Autodesk Inventor part; units mm, degrees
ref_plane "Work Plane1" through (90, 0, 0) normal (1, 0, 0) x (0, 1, 0)
ref_plane "Work Plane2" through (0, 0, 90) normal (0, 0, 1) x (1, 0, 0)
ref_plane "XZ Plane" through (0, 0, 0) normal (0, 1, 0) x (-1, 0, 0)
sketch "Sketch1" plane through (0, 0, 0) normal (0, 1, 0) x (-1, 0, 0)
  circle A0 centre (0, 0) radius 90
  dimension "d0" = 180
extrude "Extrusion1" add sketch "Sketch1" along normal blind 25
sketch "Sketch2" plane through (0, 25, 0) normal (0, 1, 0) x (1, 0, 0)
  line L0 (-30.75, 30.75) -> (30.75, 30.75)
  line L1 (30.75, 30.75) -> (30.75, -30.75)
  line L2 (30.75, -30.75) -> (-30.75, -30.75)
  line L3 (-30.75, -30.75) -> (-30.75, 30.75)
  point P0 (0, 0)
  dimension "d3" = 61.5
  dimension "d4" = 61.5
  dimension "d5" = 30.75
  dimension "d6" = 30.75
extrude "Extrusion2" cut sketch "Sketch2" against normal blind 25
sketch "Sketch3" plane through (-30.75, 25, 30.75) normal (1, 0, 0) x (0, 0, -1)
  circle A0 centre (46.5, -15) radius 1.95
  circle A1 centre (15, -15) radius 1.95
  line L0 (61.5, -25) -> (0, -25)
  line L1 (61.5, 0) -> (61.5, -25)
  line L2 (0, 0) -> (0, -25)
  point P0 (30.75, -25)
  dimension "d9" = 3.9
  dimension "d10" = 3.9
  dimension "d11" = 10
  dimension "d12" = 10
  dimension "d13" = 15
  dimension "d14" = 15
extrude "Extrusion3" cut sketch "Sketch3" along normal mid plane 300
sketch "Sketch4" plane through (-30.75, 25, -30.75) normal (0, 0, 1) x (1, 0, 0)
  circle A0 centre (30, -15) radius 1.95
  line L0 (61.5, -25) -> (0, -25)
  line L1 (0, 0) -> (0, -25)
  point P0 (30.75, -25)
  dimension "d17" = 10
  dimension "d18" = 30
  dimension "d19" = 3.9
extrude "Extrusion4" cut sketch "Sketch4" along normal mid plane 300
ref_plane "Work Plane1" through (90, 0, 0) normal (1, 0, 0) x (0, 1, 0)
sketch "Sketch5" plane through (90, 0, 0) normal (1, 0, 0) x (0, 1, 0)
  circle A0 centre (10, -15.75) radius 1.95
  circle A1 centre (10, -15.75) radius 4.5
  circle A2 centre (10, 15.75) radius 1.95
  circle A3 centre (10, 15.75) radius 4.5
  point P0 (0, 0)
  dimension "d23" = 9
  dimension "d24" = 9
extrude "Extrusion5" cut sketch "Sketch5" against normal blind 40 contours A0 | A1 | A2 | A3
mirror "Mirror1" about plane through (0, 0, 0) normal (1, 0, 0) of "Extrusion5"
ref_plane "Work Plane2" through (0, 0, 90) normal (0, 0, 1) x (1, 0, 0)
sketch "Sketch6" plane through (0, 0, 90) normal (0, 0, 1) x (1, 0, 0)
  circle A0 centre (-0.75, 10) radius 1.95
  circle A1 centre (-0.75, 10) radius 4.5
  point P0 (0, 0)
  dimension "d28" = 9
extrude "Extrusion6" cut sketch "Sketch6" against normal blind 40 contours A0 | A1
mirror "Mirror2" about plane through (0, 0, 0) normal (0, 0, 1) of "Extrusion6"
sketch "Sketch7" plane through (0, 0, 0) normal (0, -1, 0) x (1, 0, 0)
  circle A0 centre (0, 0) radius 90
  line L0 (-30.75, 30.75) -> (30.75, 30.75)
  line L1 (-30.75, 30.75) -> (30.75, 30.75)
  line L2 (30.75, 30.75) -> (30.75, -30.75)
  line L3 (30.75, -30.75) -> (-30.75, -30.75)
  line L4 (-30.75, -30.75) -> (-30.75, 30.75)
extrude "Extrusion7" add sketch "Sketch7" along normal blind 20
sketch "Sketch8" plane through (0, 25, 0) normal (0, 1, 0) x (1, 0, 0)
  line L0 (37.3786, -36.9077) -> (37.3786, 35.2103) construction
  line L1 (37.3786, 35.2103) -> (75.2405, 35.2103) construction
  line L2 (75.2405, 35.2103) -> (75.2405, -36.9077) construction
  line L3 (75.2405, -36.9077) -> (37.3786, -36.9077) construction
  point P0 (0, 0)
properties part number "Base_V2a"
Check sheet for the modelled part. Datum: model origin and axes. Units: mm. A direction names the side the tool comes from. Round coordinates to 2 decimals unless told otherwise and drop trailing zeros. Write each loop counter-clockwise with the first axis right and the second up, starting at its lowest first coordinate (ties: lowest second). Pieces come first, ordered by that corner, then holes. Notation, with made-up numbers: (87, 14) -> (120, 14) arc R33 cw to (120, 48) -> close; hole circle Ø7 at (65.5, 8.25). An arc over 180 degrees is marked (long way). Answer as CSV lines item,"result". Start each with the question number.
1) Tool access check on faces 4 (the cylindrical face through (69.922, 12.419, -11.956)), 5 (the flat face through (-50, 8, -17)), 6 (the flat face through (0, 3, -30.75)). Record the directions out of +Z, -Z, +X, -X, +Y, -Y that give a thin tool (end or side, any length) a straight path to the whole face; none if there is none.
2) Material ranges on line 1 (Z direction, x = -11.5, y = 6); line 2 (X direction, y = -1.5, z = 1.5); line 3 (Z direction, x = -59.5, y = 10), recorded low to high. Write a range as from..to.
3) Section check B-B on x = -19. Enter the section's corners in (y, z), and give its area (3 significant figures).
4) Go/stop test with flat-tipped pins: P1, Ø10, axis at y = 12, z = -16.5, coming from the -X side; P2, Ø1, axis at y = -0.5, z = 57, coming from the -X side; P3, Ø4, axis at x = -33.5, y = -3, coming from the -Z side. Record where each tip stops, or that it passes through.
5) Section check D-D on x = 60.5. Enter the section's corners in (y, z).
6) Section check A-A on y = -10. Enter the section's corners in (x, z).
7) Release check for a two-part mould opening along Y. For faces 1 (the flat face through (30.75, 3, 0)), 2 (the flat face through (-1, -20, -39)), 3 (the flat face through (50, 12, 15)) record: pulls with the +Y half, pulls with the -Y half, needs draft (parallel to the pull), parting line crosses it, or undercut.
8) Section check C-C on z = 74. Enter the section's corners in (x, y) (3 decimals), and give its area (3 significant figures).
Found:
1,face 4,"+X"
1,face 5,"-X"
1,face 6,"+Y, -Y"
2,line 1,"z = -89.26..-30.75, 30.75..89.26"
2,line 2,"x = -89.99..-30.75, 30.75..89.99"
2,line 3,"z = -67.53..-20.25, -11.25..11.25, 20.25..67.53"
3,outline,"(-20, -87.97) -> (25, -87.97) -> (25, -30.75) -> (-20, -30.75) -> close; (-20, 30.75) -> (25, 30.75) -> (25, 87.97) -> (-20, 87.97) -> close"
3,area,"5,150 mm^2"
4,P1,"stops at x = -89.26"
4,P2,"stops at x = -70.06"
4,P3,"stops at z = -84.31"
5,outline,"(-20, -66.63) -> (25, -66.63) -> (25, 66.63) -> (-20, 66.63) -> close; hole circle Ø9 at (10, -15.75); hole circle Ø9 at (10, 15.75)"
6,outline,"circle Ø180 at (0, 0); hole (-30.75, -30.75) -> (30.75, -30.75) -> (30.75, 30.75) -> (-30.75, 30.75) -> close"
7,face 1,"needs draft"
7,face 2,"pulls with the -Y half"
7,face 3,"undercut"
8,outline,"(-51.225, -20) -> (51.225, -20) -> (51.225, 25) -> (-51.225, 25) -> close; hole circle Ø9 at (-0.75, 10)"
8,area,"4,550 mm^2"
